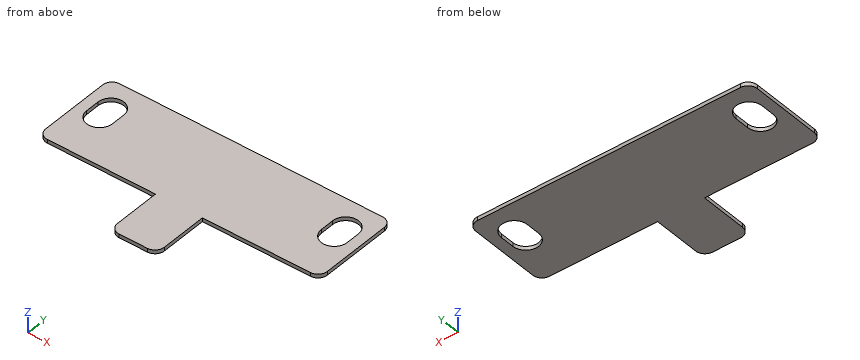
```python
from build123d import *

# Parameters (mm, degrees)
SKETCH_1_W             = 60
SKETCH_1_H             = 31
SM_BASE_FLANGE_1_DEPTH = 0.8
CUT_EXTRUDE_2_DEPTH    = 44.146726411
SKETCH_14_W            = 25
SKETCH_14_H            = 12
CUT_EXTRUDE_3_DEPTH    = 44.146726411
FILLET_3_R             = 2


# Sheet-metal steps are written as plain solids
with BuildPart() as part:
    # Sketch 1 → 基体-法兰1 (new body)
    with BuildSketch(Plane.XY):
        with Locations((0, -15.5)):
            Rectangle(SKETCH_1_W, SKETCH_1_H)
    extrude(amount=SM_BASE_FLANGE_1_DEPTH)

    # 草图13 → 切除-拉伸2 (cut, through all)
    with BuildSketch(Plane.XY.offset(0.8)):
        with BuildLine():
            Line((-27.75, -9), (-27.75, -6))
            ThreePointArc((-27.75, -6), (-25, -3.25), (-22.25, -6))
            Line((-22.25, -6), (-22.25, -9))
            ThreePointArc((-22.25, -9), (-25, -11.75), (-27.75, -9))
        make_face()
        with BuildLine():
            Line((27.75, -9), (27.75, -6))
            ThreePointArc((27.75, -6), (25, -3.25), (22.25, -6))
            Line((22.25, -6), (22.25, -9))
            ThreePointArc((22.25, -9), (25, -11.75), (27.75, -9))
        make_face()
    extrude(amount=-CUT_EXTRUDE_2_DEPTH, mode=Mode.SUBTRACT)

    # 草图14 → 切除-拉伸3 (cut, through all)
    with BuildSketch(Plane.XY.offset(0.8)):
        with Locations((-17.5, -25)):
            Rectangle(SKETCH_14_W, SKETCH_14_H)
        with Locations((17.5, -25)):
            Rectangle(SKETCH_14_W, SKETCH_14_H)
    extrude(amount=-CUT_EXTRUDE_3_DEPTH, mode=Mode.SUBTRACT)

    # 圆角3
    fillet_3_edges = [part.edges().sort_by_distance(p)[0] for p in [
        (-5, -31, 0.4),
        (-30, -19, 0.4),
        (5, -31, 0.4),
        (30, -19, 0.4),
        (-30, 0, 0.4),
        (30, 0, 0.4),
    ]]
    fillet(fillet_3_edges, radius=FILLET_3_R)


solid = part.part
```
CAD build for the part. Positions are in the model's coordinates, mm. Round coordinates to 2 decimals unless told otherwise and drop trailing zeros. Write each loop counter-clockwise with the first axis right and the second up, starting at its lowest first coordinate (ties: lowest second). Pieces come first, ordered by that corner, then holes. Notation, with made-up numbers: M 69,-24.5 L 101,-24.5 A19 cw 101,-1.5 Z; hole C 6,77.25 d1. An arc over 180 degrees is marked long. One line per question, with ' | ' between items.
1. Cut at B-B on z = 0.3. Write the cut outline in (x, y).
Working result:
outline: M -30,-17 A2 ccw -28,-19 L -5,-19 L -5,-29 A2 ccw -3,-31 L 3,-31 A2 ccw 5,-29 L 5,-19 L 28,-19 A2 ccw 30,-17 L 30,-2 A2 ccw 28,0 L -28,0 A2 ccw -30,-2 Z; hole M -27.75,-9 A2.75 ccw -22.25,-9 L -22.25,-6 A2.75 ccw -27.75,-6 Z; hole M 22.25,-9 A2.75 ccw 27.75,-9 L 27.75,-6 A2.75 ccw 22.25,-6 Z
2. Probe L1, parallel to X at y = -6.5, z = 0.25; L2, parallel to Y at x = 25, z = 0.1; L3, parallel to X at y = -3.5, z = 0.4. List the from-to ranges inside material, lowest first. Write a range as from..to.
Working result:
L1: -30..-27.75, -22.25..22.25, 27.75..30 | L2: -19..-11.75, -3.25..0 | L3: -30..-26.15, -23.85..23.85, 26.15..30
3. Cut at A-A on x = 25. Write the cut outline in (y, z), and give its area (3 significant figures).
Working result:
outline: M -19,0 L -11.75,0 L -11.75,0.8 L -19,0.8 Z; M -3.25,0 L 0,0 L 0,0.8 L -3.25,0.8 Z | area: 8.40 mm2
4. Cut at D-D on y = -23. Write the cut outline in (x, z).
Working result:
outline: M -5,0 L 5,0 L 5,0.8 L -5,0.8 Z
5. Cut at C-C on x = -11. Write the cut outline in (y, z), and give its area (3 significant figures).
Working result:
outline: M -19,0 L 0,0 L 0,0.8 L -19,0.8 Z | area: 15.2 mm2
